The listing builds one solid part. Answer for the finished solid, in the listing's coordinates (mm). Face numbers are marked on the shaded views. A direction names the side the tool comes from. Coordinates: 2 decimals unless noted, no trailing zeros. Order: outer loops, then holes, each group sorted by start corner. A loop starts at its lowest first (then second) coordinate and runs counter-clockwise, first axis right, second up. Notation, with made-up numbers: (-5.75, 32) -> (34.25, 32) arc R16 cw to (34.25, 50) -> close; hole circle Ø6 at (-17.5, 24.5). An arc over 180 degrees is marked (long way). One line per question, with ' | ' between items.
from build123d import *

# Parameters (mm, degrees)
SKETCH_1_W             = 120
SKETCH_1_H             = 50
EXTRUDE_1_DEPTH        = 15
CUT_EXTRUDE_1_REACH    = 68.708
SKETCH_2_R             = 6
HOLE_WIZARD_M3_1_D     = 2.5
HOLE_WIZARD_M3_1_DEPTH = 5
HOLE_WIZARD_M3_1_TIP   = 0.751075774
HOLE_WIZARD_M3_2_D     = 2.5
HOLE_WIZARD_M3_2_DEPTH = 5
HOLE_WIZARD_M3_2_TIP   = 0.751075774
SKETCH_19_R            = 14
CUT_EXTRUDE_3_DEPTH    = 7


with BuildPart() as part:
    # 草图1 → 凸台-拉伸1 (new body)
    with BuildSketch(Plane.XY):
        Rectangle(SKETCH_1_W, SKETCH_1_H)
    extrude(amount=EXTRUDE_1_DEPTH)

    # 草图2 → 切除-拉伸1 (cut, up to next)
    with BuildSketch(Plane.XY.offset(15), mode=Mode.PRIVATE) as cut_extrude_1_sk1:
        with Locations((-35, 0)):
            Circle(SKETCH_2_R)
    cut_extrude_1_tool1 = extrude(cut_extrude_1_sk1.sketch, amount=-CUT_EXTRUDE_1_REACH, mode=Mode.PRIVATE) & part.part
    # 草图2 → 切除-拉伸1 (cut, up to next)
    with BuildSketch(Plane.XY.offset(15), mode=Mode.PRIVATE) as cut_extrude_1_sk2:
        with Locations((35, 0)):
            Circle(SKETCH_2_R)
    cut_extrude_1_tool2 = extrude(cut_extrude_1_sk2.sketch, amount=-CUT_EXTRUDE_1_REACH, mode=Mode.PRIVATE) & part.part
    add(cut_extrude_1_tool1.solids().sort_by_distance((-35, 0, 15))[0], mode=Mode.SUBTRACT)
    add(cut_extrude_1_tool2.solids().sort_by_distance((35, 0, 15))[0], mode=Mode.SUBTRACT)

    # M3 螺纹孔1
    with Locations(Plane(origin=(0, 25, 0), x_dir=(1, 0, 0), z_dir=(0, 1, 0))):
        with Locations((30, -7.5), (-30, -7.5)):
            Hole(HOLE_WIZARD_M3_1_D / 2, depth=HOLE_WIZARD_M3_1_DEPTH)
            with Locations((0, 0, -(HOLE_WIZARD_M3_1_DEPTH + HOLE_WIZARD_M3_1_TIP / 2))):  # 118° drill point
                Cone(0, HOLE_WIZARD_M3_1_D / 2, HOLE_WIZARD_M3_1_TIP, mode=Mode.SUBTRACT)

    # M3 螺纹孔2
    with Locations(Plane(origin=(0, -25, 0), x_dir=(-1, 0, 0), z_dir=(0, -1, 0))):
        with Locations((-30, -7.5), (30, -7.5)):
            Hole(HOLE_WIZARD_M3_2_D / 2, depth=HOLE_WIZARD_M3_2_DEPTH)
            with Locations((0, 0, -(HOLE_WIZARD_M3_2_DEPTH + HOLE_WIZARD_M3_2_TIP / 2))):  # 118° drill point
                Cone(0, HOLE_WIZARD_M3_2_D / 2, HOLE_WIZARD_M3_2_TIP, mode=Mode.SUBTRACT)

    # 草图19 → 切除-拉伸3 (cut)
    with BuildSketch(Plane.XY.offset(15)):
        with Locations((-35, 0)):
            Circle(SKETCH_19_R)
        with Locations((35, 0)):
            Circle(SKETCH_19_R)
    extrude(amount=-CUT_EXTRUDE_3_DEPTH, mode=Mode.SUBTRACT)


solid = part.part
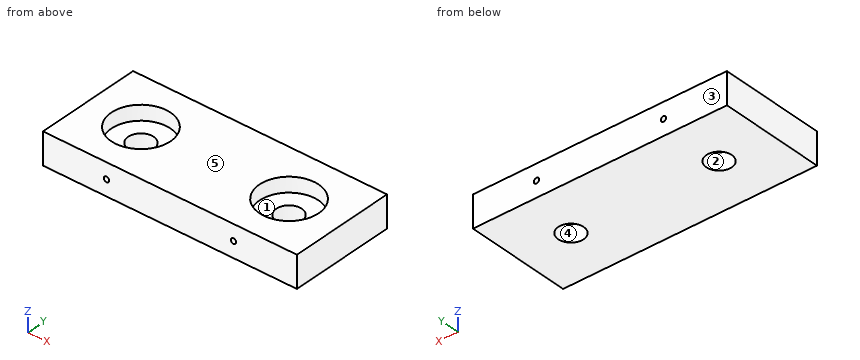
Item 1: Section D-D, the plane y = 10 is taken. Give the vertices of the cut face in (x, z).
Computed values:
outline: (-60, 0) -> (60, 0) -> (60, 15) -> (44.8, 15) -> (44.8, 8) -> (25.2, 8) -> (25.2, 15) -> (-25.2, 15) -> (-25.2, 8) -> (-44.8, 8) -> (-44.8, 15) -> (-60, 15) -> close
Item 2: Section C-C, the plane z = 13.75 is taken. Give the vertices of the cut face in (x, y), plus the area to 3 significant figures.
Computed values:
outline: (-60, -25) -> (60, -25) -> (60, 25) -> (-60, 25) -> close; hole circle Ø28 at (-35, 0); hole circle Ø28 at (35, 0) | area: 4,770 mm^2
Item 3: Section A-A, the plane y = 0 is taken. Give the vertices of the cut face in (x, z).
Computed values:
outline: (-60, 0) -> (-41, 0) -> (-41, 8) -> (-49, 8) -> (-49, 15) -> (-60, 15) -> close; (-29, 0) -> (29, 0) -> (29, 8) -> (21, 8) -> (21, 15) -> (-21, 15) -> (-21, 8) -> (-29, 8) -> close; (41, 0) -> (60, 0) -> (60, 15) -> (49, 15) -> (49, 8) -> (41, 8) -> close
Item 4: Find the intervals of material crossed by L1, parallel to X at y = -23, z = 7.5; L2, parallel to Y at x = -35, z = 5.75; L3, parallel to Y at x = 35, z = 12.5, in increasing order.
Computed values:
L1: x = -60 to -31.25, -28.75 to 28.75, 31.25 to 60 | L2: y = -25 to -6, 6 to 25 | L3: y = -25 to -14, 14 to 25
Item 5: Section B-B, the plane x = -35 is taken. Give the vertices of the cut face in (y, z), plus the area to 3 significant figures.
Computed values:
outline: (-25, 0) -> (-6, 0) -> (-6, 8) -> (-14, 8) -> (-14, 15) -> (-25, 15) -> close; (6, 0) -> (25, 0) -> (25, 15) -> (14, 15) -> (14, 8) -> (6, 8) -> close | area: 458 mm^2
Item 6: Determine the mould class of the marked faces 3, 4 and 5 for opening direction Y: pulls with the +Y half, pulls with the -Y half, needs draft (parallel to the pull), parting line crosses it, or undercut.
Computed values:
face 3: pulls with the +Y half | face 4: undercut | face 5: needs draft
Item 7: Each of these flat-tipped pins is pushed along its axis until it touches: pin 1 Ø3 at (x, z) = (-30, 7.5) entering from -Y; pin 2 Ø8.5 at (x, y) = (-39, 1) entering from +Z; pin 3 Ø1.5 at (x, z) = (-30, 7.5) entering from -Y; pin 4 Ø2 at (x, z) = (30, 7.5) entering from +Y. Where does it stop, or does it pass through?
Computed values:
pin 1: stops at y = -25 | pin 2: stops at z = 8 | pin 3: stops at y = -19.7 | pin 4: stops at y = 19.85
Item 8: For the marked faces 1 and 2, determine the directions among +Z, -Z, +X, -X, +Y, -Y from which every point of the face is accessible in a straight line to the end or side of a thin tool.
Computed values:
face 1: +Z | face 2: +Z, -Z
